Autodesk Inventor part; units mm, degrees
ref_plane "YZ Plane" through (0, 0, 0) normal (1, 0, 0) x (0, 1, 0)
ref_plane "XZ Plane" through (0, 0, 0) normal (0, 1, 0) x (-1, 0, 0)
ref_plane "XY Plane" through (0, 0, 0) normal (0, 0, 1) x (1, 0, 0)
sketch "スケッチ1" plane through (0, 0, 0) normal (0, 0, 1) x (1, 0, 0)
  line L0 (0, 0) -> (64, 0)
  line L1 (64, 0) -> (64, 64)
  line L2 (64, 64) -> (0, 64)
  line L3 (0, 64) -> (0, 0)
  line L4 (5.5, 58.5) -> (58.5, 58.5) construction
  line L5 (58.5, 58.5) -> (58.5, 5.5) construction
  line L6 (58.5, 5.5) -> (5.5, 5.5) construction
  line L7 (5.5, 5.5) -> (5.5, 58.5) construction
  circle A0 centre (5.5, 58.5) radius 1.75
  circle A1 centre (5.5, 5.5) radius 1.75
  circle A2 centre (58.5, 5.5) radius 1.75
  circle A3 centre (58.5, 58.5) radius 1.75
  line L8 (0, 32) -> (64, 32) construction
  line L9 (32, 64) -> (32, 0) construction
  line L10 (17.1, 27.05) -> (46.9, 27.05) construction
  line L11 (46.9, 27.05) -> (46.9, 36.95) construction
  line L12 (46.9, 36.95) -> (17.1, 36.95) construction
  line L13 (17.1, 36.95) -> (17.1, 27.05) construction
  line L14 (17.1, 27.05) -> (46.9, 36.95) construction
  line L15 (46.9, 27.05) -> (17.1, 36.95) construction
  circle A4 centre (46.9, 36.95) radius 1.75
  circle A5 centre (46.9, 27.05) radius 1.75
  circle A6 centre (17.1, 27.05) radius 1.75
  circle A7 centre (17.1, 36.95) radius 1.75
  point P0 (32, 32)
  dimension "d0" = 64
  dimension "d2" = 53
  dimension "d3" = 3.5
  dimension "d4" = 3.5
  dimension "d5" = 9.9
  dimension "d6" = 29.8
extrude "押し出し1" add sketch "スケッチ1" along normal blind 3
fillet "フィレット1" radius 2 4 edges at (0, 0, 1.5) (64, 0, 1.5) (64, 64, 1.5) (0, 64, 1.5)
sketch "スケッチ2" plane through (0, 0, 3) normal (0, 0, 1) x (1, 0, 0)
  circle A0 centre (17.1, 36.95) radius 1.75
  circle A1 centre (17.1, 27.05) radius 1.75
  line L0 (17.1, 36.95) -> (17.1, 27.05) construction
  line L1 (7.1, 36.95) -> (7.1, 27.05)
  line L2 (27.1, 27.05) -> (27.1, 36.95)
  arc A2 (27.1, 36.95) -> (7.1, 36.95) centre (17.1, 36.95) ccw
  arc A3 (7.1, 27.05) -> (27.1, 27.05) centre (17.1, 27.05) ccw
  circle A4 centre (46.9, 36.95) radius 1.75
  circle A5 centre (46.9, 27.05) radius 1.75
  line L3 (46.9, 36.95) -> (46.9, 27.05) construction
  line L4 (36.9, 36.95) -> (36.9, 27.05)
  line L5 (56.9, 27.05) -> (56.9, 36.95)
  arc A6 (56.9, 36.95) -> (36.9, 36.95) centre (46.9, 36.95) ccw
  arc A7 (36.9, 27.05) -> (56.9, 27.05) centre (46.9, 27.05) ccw
  point P0 (0, 0)
  point P1 (17.1, 32)
  point P2 (46.9, 32)
  dimension "d10" = 10
  dimension "d11" = 10
extrude "押し出し2" cut sketch "スケッチ2" against normal blind 0.5
properties part number "_3D プリント"
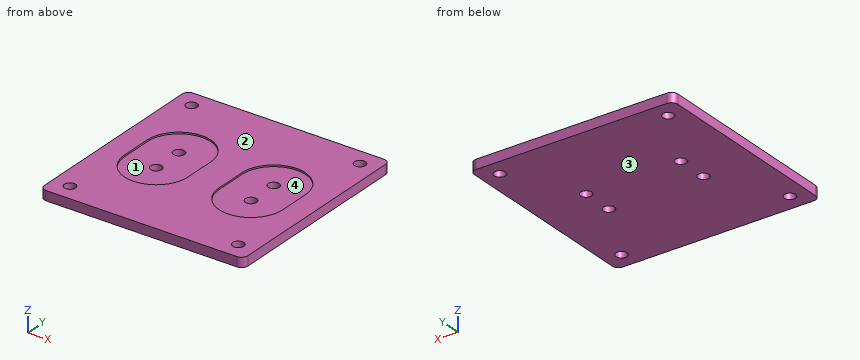
Geometry check sheet. Reference: the model listing, model coordinates, mm. Face numbers are marked on the shaded views. A direction names the side the tool comes from. Give positions to 0.01 mm unless a question says otherwise; leave off trailing zeros. Loops run counter-clockwise (first coordinate to the right, second up) from the corner with the lowest first, then second, coordinate; pieces in that order, holes last.
(1) Section check D-D on x = 17.1. Record the cut outline in (y, z), then the cut area to 3 significant figures.
From the geometry:
outline: (0, 0) - (25.3, 0) - (25.3, 2.5) - (17.05, 2.5) - (17.05, 3) - (0, 3) - close; (28.8, 0) - (35.2, 0) - (35.2, 2.5) - (28.8, 2.5) - close; (38.7, 0) - (64, 0) - (64, 3) - (46.95, 3) - (46.95, 2.5) - (38.7, 2.5) - close
area: 160 mm2
(2) Section check C-C on y = 31. Record the cut outline in (x, z).
From the geometry:
outline: (0, 0) - (64, 0) - (64, 3) - (56.9, 3) - (56.9, 2.5) - (36.9, 2.5) - (36.9, 3) - (27.1, 3) - (27.1, 2.5) - (7.1, 2.5) - (7.1, 3) - (0, 3) - close
(3) Section check B-B on z = 1.5. Count the separate pieces of the cut face and the enclosed holes in it, then the cut area to 3 significant figures.
From the geometry:
separate pieces: 1
enclosed holes: 8
area: 4,020 mm2
(4) Release check for a two-part mould opening along Y. For the marked faces 1 and 2 record: released by +Y, released by -Y, zero draft, split by the parting line, or undercut.
From the geometry:
face 1: undercut
face 2: zero draft
(5) Depth check by flat-ended pin: pin 1 Ø10 at (x, y) = (19.5, 37.5) entering from +Z; pin 2 Ø8 at (x, y) = (8.5, 21.5) entering from -Z. Enter the tip coordinate at first touch or a pass-through.
From the geometry:
pin 1: stops at z = 2.5
pin 2: stops at z = 0
(6) Set-up check for the marked faces 3 and 4: record each of +Z, -Z, +X, -X, +Y, -Y from which the full face is reachable in a straight line by a thin tool's end or side.
From the geometry:
face 3: -Z, +X, -X, +Y, -Y
face 4: +Z
(7) Thickness scan on L1, parallel to Y at x = 17.1, z = 0.85; L2, parallel to Y at x = 5.5, z = 1.85; L3, parallel to X at y = 4, z = 1.2. Record the ranges inside material, lowest first.
From the geometry:
L1: y = 0 to 25.3, 28.8 to 35.2, 38.7 to 64
L2: y = 0 to 3.75, 7.25 to 56.75, 60.25 to 64
L3: x = 0 to 4.6, 6.4 to 57.6, 59.4 to 64
(8) Section check A-A on x = 58.5. Record the cut outline in (y, z), then the cut area to 3 significant figures.
From the geometry:
outline: (0, 0) - (3.75, 0) - (3.75, 3) - (0, 3) - close; (7.25, 0) - (56.75, 0) - (56.75, 3) - (7.25, 3) - close; (60.25, 0) - (64, 0) - (64, 3) - (60.25, 3) - close
area: 171 mm2
